Here's how the part is built. I have some questions about the finished solid (model axes, mm). A direction names the side the tool comes from. Round coordinates to 2 decimals unless told otherwise and drop trailing zeros. Loops run counter-clockwise (first coordinate to the right, second up) from the corner with the lowest first, then second, coordinate; pieces in that order, holes last. Notation, with made-up numbers: M 56,-2 L 97,-2 A24 ccw 97,12 Z; hole C 86.5,78 d4. An arc over 180 degrees is marked long. Answer as a JSON object with one key per item and string values.
from build123d import *

# Parameters (mm, degrees)
BOSS_EXTRUDE1_DEPTH       = 6.35
TAP_DRILL_FOR_4_40_TAP1_D = 2.2606


with BuildPart() as part:
    # Sketch2 → Boss-Extrude1 (new body)
    with BuildSketch(Plane.YZ):
        with BuildLine():
            Line((-6.35, -10.998522628), (-6.35, -18.618522628))
            Line((-6.35, -18.618522628), (-7.9375, -18.618522628))
            Line((-7.9375, -18.618522628), (-7.9375, -11.879762203))
            ThreePointArc((-7.9375, -11.879762203), (0, 14.2875), (7.9375, -11.879762203))
            Line((7.9375, -11.879762203), (7.9375, -18.618522628))
            Line((7.9375, -18.618522628), (6.35, -18.618522628))
            Line((6.35, -18.618522628), (6.35, -10.998522628))
            ThreePointArc((6.35, -10.998522628), (0, 12.7), (-6.35, -10.998522628))
        make_face()
    extrude(amount=BOSS_EXTRUDE1_DEPTH)

    # Tap Drill for #4-40 Tap1 (through all)
    with Locations(Plane.XZ.offset(7.9375)):
        with Locations((3.175, -16.237272628)):
            Hole(TAP_DRILL_FOR_4_40_TAP1_D / 2)


solid = part.part
Item 1: If I drill on L1, parallel to Y at x = 3.5, z = -13.5; L2, parallel to Z at x = 3.75, y = 6.5; L3, parallel to Y at x = 4.5, z = -2, over which ranges is the centre line in solid material (lowest first)? Write a range as from..to.
Solution:
{"L1": "y = -7.94..-6.35, 6.35..7.94", "L2": "z = -18.62..-17.21, -15.26..-10.91, 10.91..12.72", "L3": "y = -14.15..-12.54, 12.54..14.15"}
Item 2: I want a section at A-A on z = 0. List the corners of the cut face in (x, y) for me.
Solution:
{"outline": "M 0,-14.29 L 6.35,-14.29 L 6.35,-12.7 L 0,-12.7 Z; M 0,12.7 L 6.35,12.7 L 6.35,14.29 L 0,14.29 Z"}
Item 3: For faces 1 (the face through (3, 7, -18.619)), 2 (the face through (3.1, -7.938, -14.5)), 3 (the face through (3.1, -6.35, -14.8)), 4 (the face through (3, 7.938, -14)), which set-ups out of +Z, -Z, +X, -X, +Y, -Y let a thin tool reach every point of the face, with its end or its side?
Solution:
{"face 1": "-Z, +X, -X, +Y, -Y", "face 2": "-Z, +X, -X, -Y", "face 3": "-Z, +X, -X", "face 4": "-Z, +X, -X, +Y"}
Item 4: We'd pull the mould along Y, two halves only. Please class faces 5 (the face through (0, 11, -7)), 6 (the face through (3.13, -0.51, 14.28)), 7 (the face through (3.13, 0.47, 12.69)): +Y half, -Y half, draft (parallel to the pull), parting line (faces both ways), or undercut.
Solution:
{"face 5": "draft", "face 6": "parting line", "face 7": "undercut"}
Item 5: I want a section at C-C on y = 0. List the corners of the cut face in (x, z) for me, plus the area to 3 significant figures.
Solution:
{"outline": "M 0,12.7 L 6.35,12.7 L 6.35,14.29 L 0,14.29 Z", "area": "10.1 mm2"}
Item 6: I want a section at D-D on z = -6. List the corners of the cut face in (x, y) for me.
Solution:
{"outline": "M 0,-12.97 L 6.35,-12.97 L 6.35,-11.19 L 0,-11.19 Z; M 0,11.19 L 6.35,11.19 L 6.35,12.97 L 0,12.97 Z"}
Item 7: For P1, Ø3.5, axis at x = 3.18, z = -16.24, coming from the -Y side; P2, Ø2.5, axis at x = 3.18, z = -16.24, coming from the +Y side; P3, Ø1, axis at x = 4.5, y = -11, coming from the -Z side, each with a flat end and sliding along its axis, tell me the tip position at first contact or that it passes through.
Solution:
{"P1": "stops at y = -7.94", "P2": "stops at y = 7.94", "P3": "stops at z = -9.69"}
